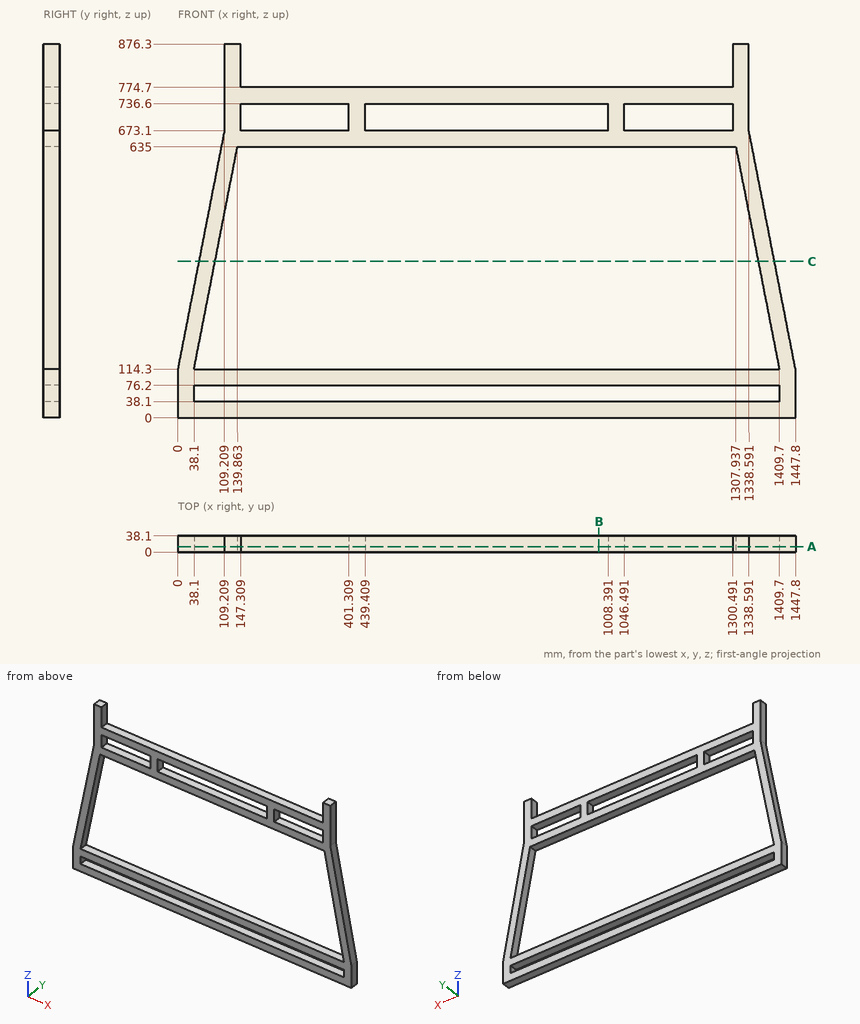
Could you check a few things on this drawing? It's one solid part, dimensions in mm from its lowest x, y, z. Give positions to 0.01 mm unless a question says otherwise; leave off trailing zeros. Order: outer loops, then holes, each group sorted by start corner. A loop starts at its lowest first (then second) coordinate and runs counter-clockwise, first axis right, second up.
1. Suppose I cut it at A-A (y = 13). State how many separate pieces and enclosed holes the cut face has, plus the area to 3 significant figures.
Answers below:
separate pieces: 1
enclosed holes: 5
area: 264,000 mm2
2. For pin 1 (11.5 mm diameter, centred on x = 1123.5, y = 26, fed in from +Z); pin 2 (11.5 mm diameter, centred on y = 20, z = 715, fed in from +X); pin 3 (3 mm diameter, centred on y = 21, z = 141, fed in from +X) (3 decimals), each with a flat end and sliding along its axis, tell me the tip position at first contact or that it passes through.
Answers below:
pin 1: stops at z = 774.7
pin 2: stops at x = 1338.59
pin 3: stops at x = 1442.875
3. Suppose I cut it at C-C (z = 367). Write out the boundary of the cut face in (x, y), plus the area to 3 significant figures.
Answers below:
outline: (49.39, 0) - (87.49, 0) - (87.49, 38.1) - (49.39, 38.1) - close; (1360.31, 0) - (1398.41, 0) - (1398.41, 38.1) - (1360.31, 38.1) - close
area: 2,900 mm2
4. I need wall thicknesses on L1, parallel to Z at x = 231.5, y = 27.5; L2, parallel to X at y = 13, z = 728.5; L3, parallel to Z at x = 410.5, y = 36. Which ranges of each line are inside material? Lowest first, please.
Answers below:
L1: z = 0 to 38.1, 76.2 to 114.3, 635 to 673.1, 736.6 to 774.7
L2: x = 109.21 to 147.31, 401.31 to 439.41, 1008.39 to 1046.49, 1300.49 to 1338.59
L3: z = 0 to 38.1, 76.2 to 114.3, 635 to 774.7
5. Suppose I cut it at B-B (x = 987). Write out the boundary of the cut face in (y, z).
Answers below:
outline: (0, 0) - (38.1, 0) - (38.1, 38.1) - (0, 38.1) - close; (0, 76.2) - (38.1, 76.2) - (38.1, 114.3) - (0, 114.3) - close; (0, 635) - (38.1, 635) - (38.1, 673.1) - (0, 673.1) - close; (0, 736.6) - (38.1, 736.6) - (38.1, 774.7) - (0, 774.7) - close
